Design review of the part built by this model. Coordinates are the model's own, in mm. Face numbers are marked on the shaded views. A direction names the side the tool comes from. Coordinates: 2 decimals unless noted, no trailing zeros. Write each loop counter-clockwise with the first axis right and the second up, starting at its lowest first coordinate (ties: lowest second). Pieces come first, ordered by that corner, then holes.
Q1. Insertion check: pin 1 (2.5 mm diameter, centred on y = -18, z = 2, fed in from +X); pin 2 (1.5 mm diameter, centred on x = -7.5, z = 3.5, fed in from -Y); pin 3 (2.5 mm diameter, centred on y = -18.5, z = 3.5, fed in from -X). Each pin has a flat end and moves straight along its axis. Give the tip position at first contact, or say it passes through.
Q2. For probe 1 along Y at (x, z) = (0, 2.3); probe 2 along X at (y, z) = (-16, 2.6); probe 3 along Y at (x, z) = (8, 3.8), list the stretches that pass through material, from the lowest coordinate up.
Q3. Take a section at C-C (y = -29). Give the boundary of the cut face in (x, z), and give its area (3 significant figures).
Q4. Take a section at A-A (x = 0). Give the boundary of the cut face in (y, z), and give its area (3 significant figures).
Q5. Take a section at D-D (y = -5.5). Give the boundary of the cut face in (x, z), and give its area (3 significant figures).
Q6. Mouldability with a two-part tool opening along Y and no side actions: class the marked faces 1, 2, 3 and 4 as pulls with the +Y half, pulls with the -Y half, needs draft (parallel to the pull), parting line crosses it, or undercut.
Q7. Take a section at B-B (z = 1.6). Give the boundary of the cut face in (x, y).
Q8. Machinability: for the marked faces 5, 6 and 7, which of the approach directions +Z, -Z, +X, -X, +Y, -Y give a long, thin tool a straight path to every point of the face, cutting with its end or side? Answer none if there is none.
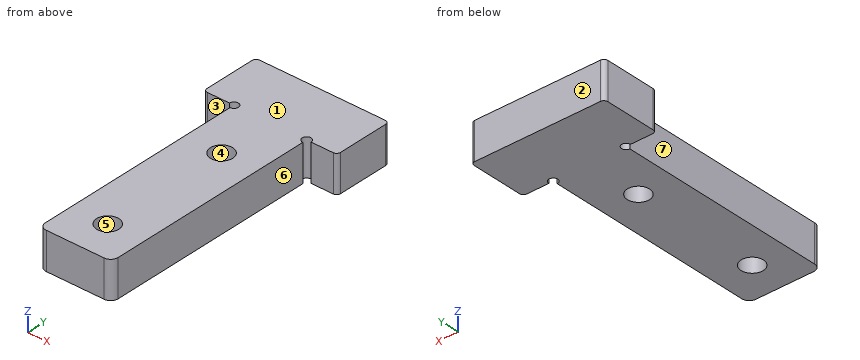
```python
from build123d import *

# Parameters (mm, degrees)
SKETCH_1_R      = 1.5
EXTRUDE_1_DEPTH = 5


with BuildPart() as part:
    # 草图1 → 凸台-拉伸1 (new body)
    with BuildSketch(Plane.XY):
        with BuildLine():
            Line((-4.9, -4.6), (-4.9, -33))
            ThreePointArc((-4.9, -33), (-4.607106781, -33.707106781), (-3.9, -34))
            Line((-3.9, -34), (3.9, -34))
            ThreePointArc((3.9, -34), (4.607106781, -33.707106781), (4.9, -33))
            Line((4.9, -33), (4.9, -4.6))
            ThreePointArc((4.9, -4.6), (4.475735931, -3.575735931), (5.5, -4))
            Line((5.5, -4), (5.9, -4))
            Line((5.9, -4), (8.480562012, -4))
            ThreePointArc((8.480562012, -4), (8.847860136, -3.847860136), (9, -3.480562012))
            Line((9, -3.480562012), (9, 3.480562012))
            ThreePointArc((9, 3.480562012), (8.847860136, 3.847860136), (8.480562012, 4))
            Line((8.480562012, 4), (-8.480562012, 4))
            ThreePointArc((-8.480562012, 4), (-8.847860136, 3.847860136), (-9, 3.480562012))
            Line((-9, 3.480562012), (-9, -3.480562012))
            ThreePointArc((-9, -3.480562012), (-8.847860136, -3.847860136), (-8.480562012, -4))
            Line((-8.480562012, -4), (-5.9, -4))
            Line((-5.9, -4), (-5.5, -4))
            ThreePointArc((-5.5, -4), (-4.475735931, -3.575735931), (-4.9, -4.6))
        make_face()
        with Locations((0, -11.5)):
            Circle(SKETCH_1_R, mode=Mode.SUBTRACT)
        with Locations((0, -29)):
            Circle(SKETCH_1_R, mode=Mode.SUBTRACT)
    extrude(amount=EXTRUDE_1_DEPTH)


solid = part.part
```
Response:
1. pin 1: stops at x = 4.9
1. pin 2: stops at y = -4
1. pin 3: stops at x = -4.9
2. probe 1: y = -34 to -30.5, -27.5 to -13, -10 to 4
2. probe 2: x = -4.9 to 4.9
2. probe 3: y = -4 to 4
3. outline: (-4.9, 0) - (-1.5, 0) - (-1.5, 5) - (-4.9, 5) - close; (1.5, 0) - (4.9, 0) - (4.9, 5) - (1.5, 5) - close
3. area: 34.0 mm2
4. outline: (-34, 0) - (-30.5, 0) - (-30.5, 5) - (-34, 5) - close; (-27.5, 0) - (-13, 0) - (-13, 5) - (-27.5, 5) - close; (-10, 0) - (4, 0) - (4, 5) - (-10, 5) - close
4. area: 160 mm2
5. outline: (-4.9, 0) - (4.9, 0) - (4.9, 5) - (-4.9, 5) - close
5. area: 49.0 mm2
6. face 1: needs draft
6. face 2: pulls with the +Y half
6. face 3: pulls with the -Y half
6. face 4: undercut
7. outline: (-9, -3.48) arc R0.52 ccw to (-8.48, -4) - (-5.5, -4) arc R0.6 cw (long way) to (-4.9, -4.6) - (-4.9, -33) arc R1 ccw to (-3.9, -34) - (3.9, -34) arc R1 ccw to (4.9, -33) - (4.9, -4.6) arc R0.6 cw (long way) to (5.5, -4) - (8.48, -4) arc R0.52 ccw to (9, -3.48) - (9, 3.48) arc R0.52 ccw to (8.48, 4) - (-8.48, 4) arc R0.52 ccw to (-9, 3.48) - close; hole circle Ø3 at (0, -29); hole circle Ø3 at (0, -11.5)
8. face 5: +Z, -Z
8. face 6: +Z, -Z, +X, -Y
8. face 7: +Z, -Z, -X, -Y
